Build history of the part. All positions in model axes, mm. Face numbers are marked on the shaded views. A direction names the side the tool comes from. Give positions to 0.01 mm unless a question says otherwise; leave off trailing zeros. Write each loop counter-clockwise with the first axis right and the second up, starting at its lowest first coordinate (ties: lowest second). Pieces come first, ordered by that corner, then holes.
from build123d import *
from build123d.topology import SkipClean

# Parameters (mm, degrees)
SKETCH_1_W          = 30
SKETCH_1_H          = 30
SKETCH_1_R          = 10.5
EXTRUDE_1_DEPTH     = 17
SKETCH_2_W          = 30
SKETCH_2_H          = 30
EXTRUDE_2_DEPTH     = 25
SKETCH_3_R          = 0.95
CUT_EXTRUDE_1_DEPTH = 54.749418602
SKETCH_4_R          = 2.5
CUT_EXTRUDE_2_DEPTH = 2
CUT_EXTRUDE_START   = -2
SKETCH_5_R          = 2.5
CUT_EXTRUDE_3_DEPTH = 2
SKETCH_6_W          = 19
SKETCH_6_H          = 10
EXTRUDE_5_DEPTH     = 20
SKETCH_8_W          = 19
SKETCH_8_H          = 10
EXTRUDE_6_DEPTH     = 20
SKETCH_9_R          = 3
CUT_EXTRUDE_4_DEPTH = 10
SKETCH_10_R         = 4.5
CUT_EXTRUDE_5_DEPTH = 6


with BuildPart() as part:
    # 草图1 → 凸台-拉伸1 (new body)
    with BuildSketch(Plane.XY):
        Rectangle(SKETCH_1_W, SKETCH_1_H)
        Circle(SKETCH_1_R, mode=Mode.SUBTRACT)
    extrude(amount=EXTRUDE_1_DEPTH)

    # 草图2 → 凸台-拉伸2 (add)
    with SkipClean():  # the faces are left unmerged after this step: merging them gives an invalid solid
        with BuildSketch(Plane.XY.offset(17)):
            Rectangle(SKETCH_2_W, SKETCH_2_H)
            with BuildLine():
                Line((-6.800735254, 8), (6.800735254, 8))
                ThreePointArc((6.800735254, 8), (10.5, 0), (6.800735254, -8))
                Line((6.800735254, -8), (-6.800735254, -8))
                ThreePointArc((-6.800735254, -8), (-10.5, 0), (-6.800735254, 8))
            make_face(mode=Mode.SUBTRACT)
        extrude(amount=EXTRUDE_2_DEPTH)

    # 草图3 → 切除-拉伸1 (cut, through all)
    with SkipClean():  # the faces are left unmerged after this step: merging them gives an invalid solid
        with BuildSketch(Plane(origin=(0, 15, 0), x_dir=(1, 0, 0), z_dir=(0, 1, 0))):
            with Locations(Location((0, -34, 0), (0, 0, 270))):
                Circle(SKETCH_3_R)
            with Locations(Location((0, -8, 0), (0, 0, 270))):
                Circle(SKETCH_3_R)
            with Locations(Location((0, -24, 0), (0, 0, 270))):
                Circle(SKETCH_3_R)
        extrude(amount=-CUT_EXTRUDE_1_DEPTH, mode=Mode.SUBTRACT)

    # 草图4 → 切除-拉伸2 (cut)
    with SkipClean():  # the faces are left unmerged after this step: merging them gives an invalid solid
        with BuildSketch(Plane(origin=(0, 15, 0), x_dir=(1, 0, 0), z_dir=(0, 1, 0))):
            with Locations(Location((0, -8, 0), (0, 0, 270))):
                Circle(SKETCH_4_R)
            with Locations(Location((0, -24, 0), (0, 0, 270))):
                Circle(SKETCH_4_R)
            with Locations(Location((0, -34, 0), (0, 0, 270))):
                Circle(SKETCH_4_R)
        extrude(amount=-CUT_EXTRUDE_2_DEPTH, mode=Mode.SUBTRACT)

    # 草图5 → 切除-拉伸3 (cut)
    with SkipClean():  # the faces are left unmerged after this step: merging them gives an invalid solid
        with BuildSketch(Plane.XZ.offset(15).offset(CUT_EXTRUDE_START)):
            with Locations(Location((0, 34, 0), (0, 0, 90))):
                Circle(SKETCH_5_R)
            with Locations(Location((0, 24, 0), (0, 0, 90))):
                Circle(SKETCH_5_R)
            with Locations(Location((0, 8, 0), (0, 0, 90))):
                Circle(SKETCH_5_R)
        extrude(amount=CUT_EXTRUDE_3_DEPTH, mode=Mode.SUBTRACT)

    # 草图6 → 凸台-拉伸5 (add)
    with SkipClean():  # the faces are left unmerged after this step: merging them gives an invalid solid
        with BuildSketch(Plane.ZY.offset(15)):
            with Locations((18.5, 10)):
                Rectangle(SKETCH_6_W, SKETCH_6_H)
        extrude(amount=EXTRUDE_5_DEPTH)

    # 草图8 → 凸台-拉伸6 (add)
    with SkipClean():  # the faces are left unmerged after this step: merging them gives an invalid solid
        with BuildSketch(Plane(origin=(15, 0, 0), x_dir=(0, 0, -1), z_dir=(1, 0, 0))):
            with Locations((-18.5, 10)):
                Rectangle(SKETCH_8_W, SKETCH_8_H)
        extrude(amount=EXTRUDE_6_DEPTH)

    # 草图9 → 切除-拉伸4 (cut)
    with SkipClean():  # the faces are left unmerged after this step: merging them gives an invalid solid
        with BuildSketch(Plane.XZ.offset(-5)):
            with Locations(Location((-25, 19, 0), (0, 0, 270))):
                Circle(SKETCH_9_R)
            with Locations(Location((25, 19, 0), (0, 0, 270))):
                Circle(SKETCH_9_R)
        extrude(amount=-CUT_EXTRUDE_4_DEPTH, mode=Mode.SUBTRACT)

    # 草图10 → 切除-拉伸5 (cut)
    with SkipClean():  # the faces are left unmerged after this step: merging them gives an invalid solid
        with BuildSketch(Plane.XZ.offset(-5)):
            with Locations(Location((-25, 19, 0), (0, 0, 270))):
                Circle(SKETCH_10_R)
            with Locations(Location((25, 19, 0), (0, 0, 270))):
                Circle(SKETCH_10_R)
        extrude(amount=-CUT_EXTRUDE_5_DEPTH, mode=Mode.SUBTRACT)


solid = part.part
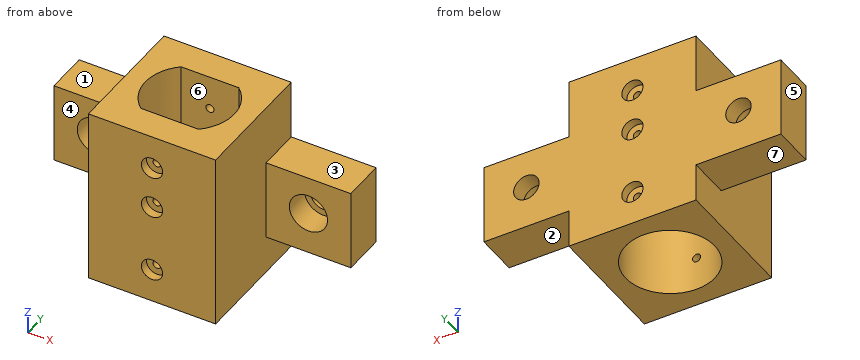
(1) 3-axis set-ups, long thin cutter, end or side, ignore diameter. For the marked faces 1, 2, 3 and 4: which of +Z, -Z, +X, -X, +Y, -Y reach the whole face in a straight line?
(2) Probe line 1 (X direction, y = -14, z = 34); line 2 (X direction, y = 0.5, z = 7); line 3 (Y direction, x = 0, z = 13.25). List the from-to ranges inside material, lowest first.
(3) Saw through at B-B, the plane y = 0. List the corners of the cut face in (x, z), plus the area to 3 significant figures.
(4) Saw through at C-C, the plane x = -25. List the corners of the cut face in (y, z), plus the area to 3 significant figures.
(5) Saw through at A-A, the plane z = 19. List the corners of the cut face in (x, y), plus the area to 3 significant figures.
(6) Drop flat-ended pins along their axis: pin 1 (9.5 mm diameter, centred on x = -30, z = 15.5, fed in from -Y); pin 2 (4 mm diameter, centred on x = -17.5, y = 7.5, fed in from -Z); pin 3 (1.5 mm diameter, centred on x = 1, z = 35, fed in from -Y). Give the stop position or say it passes through.
(7) Mould opens along X. For the marked faces 5, 6 and 7 say: +X half, -X half, draft (parallel to the pull), parting line (faces both ways), or undercut.
(8) Saw through at D-D, the plane z = 38.5. List the corners of the cut face in (x, y).
Computed values:
1. face 1: +Z, -X, +Y, -Y
1. face 2: -Z, +X, +Y, -Y
1. face 3: +Z, +X, +Y, -Y
1. face 4: +Z, -Z, -X, -Y
2. line 1: x = -15 to -2.5, 2.5 to 15
2. line 2: x = -15 to -10.49, 10.49 to 15
2. line 3: y = -15 to -10.5, 10.5 to 15
3. outline: (-15, 0) - (-10.5, 0) - (-10.5, 42) - (-15, 42) - close; (10.5, 0) - (15, 0) - (15, 42) - (10.5, 42) - close
3. area: 378 mm2
4. outline: (5, 9) - (15, 9) - (15, 16) - (11, 16) - (11, 14.5) - (5, 14.5) - close; (5, 23.5) - (11, 23.5) - (11, 22) - (15, 22) - (15, 28) - (5, 28) - close
4. area: 112 mm2
5. outline: (-35, 5) - (-29.5, 5) - (-29.5, 11) - (-28, 11) - (-28, 15) - (-35, 15) - close; (-22, 11) - (-20.5, 11) - (-20.5, 5) - (-15, 5) - (-15, -15) - (15, -15) - (15, 5) - (20.5, 5) - (20.5, 11) - (22, 11) - (22, 15) - (-22, 15) - close; (28, 11) - (29.5, 11) - (29.5, 5) - (35, 5) - (35, 15) - (28, 15) - close; hole (-6.8, -8) - (6.8, -8) arc R10.5 ccw to (6.8, 8) - (-6.8, 8) arc R10.5 ccw to start
5. area: 844 mm2
6. pin 1: stops at y = 5
6. pin 2: stops at z = 9
6. pin 3: stops at y = -13
7. face 5: -X half
7. face 6: undercut
7. face 7: draft
8. outline: (-15, -15) - (15, -15) - (15, 15) - (-15, 15) - close; hole (-6.8, -8) - (6.8, -8) arc R10.5 ccw to (6.8, 8) - (-6.8, 8) arc R10.5 ccw to start
